Study the drawing (mm; zero at the part's minimum x, y, z) and answer. Coordinates: 2 decimals unless noted, no trailing zeros. Loops run counter-clockwise (first coordinate to the right, second up) from the corner with the lowest first, then second, coordinate; pieces in that order, holes last.
Q1. Straight lines are drawn through the part: line 1 (X direction, y = 60, z = 2.3) (1 decimal); line 2 (Y direction, x = 61, z = 0.45) (1 decimal); line 3 (X direction, y = 11, z = 2.85) (1 decimal). For each, find the intervals that lie inside material, in ascending order.
Q2. Section A-A (y = 40) is taken. Give the vertices of the cut face in (x, z), then the cut area to 3 significant figures.
Q3. Flat-ended cylindrical pins translate along their axes: P1, Ø1.5, axis at x = 42.5, z = 1, coming from the +Y side; P2, Ø1.5, axis at x = 47.5, z = 2.5, coming from the -Y side (1 decimal); P3, Ø1, axis at y = 36.5, z = 2, coming from the +X side. Find the tip coordinate at first contact, or state that the pin passes through.
Q4. Section B-B (x = 62.5) is taken. Give the vertices of the cut face in (y, z) (1 decimal).
Q5. Section D-D (x = 11.5) is taken. Give the vertices of the cut face in (y, z), then the cut area to 3 significant figures.
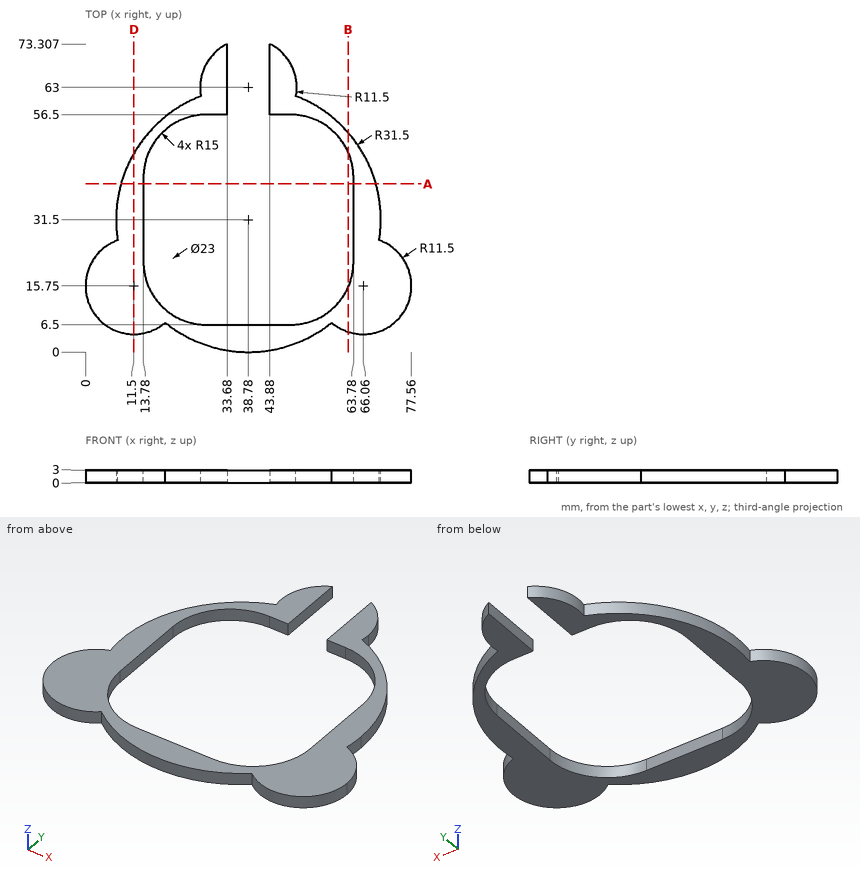
Numbers:
1. line 1: x = 25.4 to 33.7, 43.9 to 52.2
1. line 2: y = 5.4 to 12.8, 50.2 to 53.8
1. line 3: x = 1 to 18.1, 59.5 to 76.5
2. outline: (8.45, 0) - (13.78, 0) - (13.78, 3) - (8.45, 3) - close; (63.78, 0) - (69.11, 0) - (69.11, 3) - (63.78, 3) - close
2. area: 32.0 mm2
3. P1: stops at y = 6.5
3. P2: stops at y = 1
3. P3: stops at x = 69.96
4. outline: (4.8, 0) - (15.4, 0) - (15.4, 3) - (4.8, 3) - close; (47.6, 0) - (52.2, 0) - (52.2, 3) - (47.6, 3) - close
5. outline: (4.25, 0) - (47.25, 0) - (47.25, 3) - (4.25, 3) - close
5. area: 129 mm2
